CAD build for the part. Positions are in the model's coordinates, mm. Coordinates: 2 decimals unless noted, no trailing zeros. Loops run counter-clockwise (first coordinate to the right, second up) from the corner with the lowest first, then second, coordinate; pieces in that order, holes last.
1) Pin check, flat tips, straight feed: pin 1 Ø4.5 at (x, y) = (53.975, 0) entering from +Z (3 decimals); pin 2 Ø2 at (x, y) = (73.025, 0) entering from +Z; pin 3 Ø1.5 at (y, z) = (5, 4.5) entering from -X; pin 4 Ø3 at (y, z) = (-2.5, 3) entering from -X. Stop position of each tip, or through.
2) Two-plate mould, pull along Y, no slides. Class faces 1 (the flat face through (-1, 0, 0)), 2 (the flat face through (1, 9.525, 2)), 3 (the cylindrical face through (55.57, 0.5, 2.3)): +Y half, -Y half, draft (parallel to the pull), parting line (faces both ways), or undercut.
3) Saw through at A-A, the plane z = 2. Write the cut outline in (x, y) (3 decimals).
4) Saw through at B-B, the plane x = 33.5. Write the cut outline in (y, z) (3 decimals).
5) Wall check: line 1 along Y through (x, z) = (-15, 3.25); line 2 along Z through (x, y) = (66.5, -6.5); line 3 along Y through (x, z) = (72.5, 3.5). Give the ranges that are in metal, low to high.
```python
from build123d import *

# Parameters (mm, degrees)
F0_R     = 1.67
F1_DEPTH = 6.35
F2_R     = 3.175
F3_SIZE  = 1.675


with BuildPart() as f1:
    # F0 (on Top) → F1 (new body)
    with BuildSketch(Plane.XY):
        with BuildLine():
            Line((73.025, 9.525), (63.5, 9.525))
            Line((63.5, 9.525), (-63.5, 9.525))
            Line((-63.5, 9.525), (-73.025, 9.525))
            ThreePointArc((-73.025, 9.525), (-79.7601920908, 6.7351920908), (-82.55, 0))
            ThreePointArc((-82.55, 0), (-79.7601920908, -6.7351920908), (-73.025, -9.525))
            Line((-73.025, -9.525), (-63.5, -9.525))
            Line((-63.5, -9.525), (63.5, -9.525))
            Line((63.5, -9.525), (73.025, -9.525))
            ThreePointArc((73.025, -9.525), (79.7601920908, -6.7351920908), (82.55, 0))
            ThreePointArc((82.55, 0), (79.7601920908, 6.7351920908), (73.025, 9.525))
        make_face()
        with Locations((-73.025, 0)):
            Circle(F0_R, mode=Mode.SUBTRACT)
        with Locations((-53.975, 0)):
            Circle(F0_R, mode=Mode.SUBTRACT)
        with Locations((53.975, 0)):
            Circle(F0_R, mode=Mode.SUBTRACT)
        with Locations((73.025, 0)):
            Circle(F0_R, mode=Mode.SUBTRACT)
    extrude(amount=F1_DEPTH)

    # F2
    f2_edges = [f1.edges().sort_by_distance(p)[0] for p in [
        (-82.55, 0, 6.35),
        (82.55, 0, 6.35),
        (0, 9.525, 6.35),
        (0, -9.525, 6.35),
    ]]
    fillet(f2_edges, radius=F2_R)

    # F3
    f3_edges = [f1.edges().sort_by_distance(p)[0] for p in [
        (-74.695, 0, 6.35),
        (-55.645, 0, 6.35),
        (52.305, 0, 6.35),
        (71.355, 0, 6.35),
    ]]
    chamfer(f3_edges, length=F3_SIZE)


solid = f1.part
```
Data:
1. pin 1: stops at z = 5.255
1. pin 2: passes through
1. pin 3: stops at x = -81.34
1. pin 4: stops at x = -82.5
2. face 1: draft
2. face 2: +Y half
2. face 3: undercut
3. outline: (-73.025, -9.525) - (73.025, -9.525) arc R9.525 ccw to (73.025, 9.525) - (-73.025, 9.525) arc R9.525 ccw to start; hole circle Ø3.34 at (-73.025, 0); hole circle Ø3.34 at (-53.975, 0); hole circle Ø3.34 at (53.975, 0); hole circle Ø3.34 at (73.025, 0)
4. outline: (-9.525, 0) - (9.525, 0) - (9.525, 3.175) arc R3.175 ccw to (6.35, 6.35) - (-6.35, 6.35) arc R3.175 ccw to (-9.525, 3.175) - close
5. line 1: y = -9.52 to 9.52
5. line 2: z = 0 to 6.35
5. line 3: y = -9.51 to -1.59, 1.59 to 9.51
